```python
from build123d import *

# Parameters (mm, degrees)
SKETCH1_W               = 400
SKETCH1_H               = 200
BOSS_EXTRUDE1_DEPTH     = 52.5
SKETCH2_W               = 400
SKETCH2_H               = 90
CUT_EXTRUDE2_DEPTH      = 40
SKETCH3_W               = 90.375416362
SKETCH3_H               = 10.805756305
CUT_EXTRUDE4_DEPTH      = 30
SKETCH6_W               = 90.866587104
SKETCH6_H               = 12.770439269
CUT_EXTRUDE5_DEPTH      = 30
SKETCH7_W               = 90.866587104
SKETCH7_H               = 151.035002888
CUT_EXTRUDE6_DEPTH      = 416.639567414
SKETCH8_W               = 30
SKETCH8_H               = 90.375416362
CUT_EXTRUDE7_DEPTH      = 256.367226621
SKETCH11_R              = 11.25
CUT_EXTRUDE8_DEPTH      = 248.032386541
FILLET6_R               = 5
CUT_EXTRUDE9_DEPTH      = 248.032386541
CUT_EXTRUDE9_DEPTH_BACK = 248.032386541
SKETCH12_R              = 11.25
FILLET7_R               = 5
SKETCH19_W              = 5.960521718
SKETCH19_H              = 90
CUT_EXTRUDE11_DEPTH     = 262.450282081
SKETCH20_W              = 5
SKETCH20_H              = 90
CUT_EXTRUDE12_DEPTH     = 262.450282081
BOSS_EXTRUDE7_REACH     = 249.032
SKETCH29_W              = 29.604200123
SKETCH29_H              = 5.313574381
SKETCH30_W              = 40.6
SKETCH30_H              = 6.563827177
CUT_EXTRUDE16_DEPTH     = 416.639567414
SKETCH31_R              = 2.65
CUT_EXTRUDE17_DEPTH     = 10
SKETCH32_W              = 53.894825864
SKETCH32_H              = 4.174951299
BOSS_EXTRUDE8_DEPTH     = 5
SKETCH33_W              = 38.657413524
SKETCH33_H              = 4.433580482
BOSS_EXTRUDE9_DEPTH     = 5


with BuildPart() as part:
    # Sketch1 → Boss-Extrude1 (new, symmetric)
    with BuildSketch(Plane.XY):
        Rectangle(SKETCH1_W, SKETCH1_H)
    extrude(amount=BOSS_EXTRUDE1_DEPTH, both=True)

    # Sketch2 → Cut-Extrude2 (cut)
    with BuildSketch(Plane(origin=(0, 100, 0), x_dir=(1, 0, 0), z_dir=(0, 1, 0))):
        Rectangle(SKETCH2_W, SKETCH2_H)
    extrude(amount=-CUT_EXTRUDE2_DEPTH, mode=Mode.SUBTRACT)

    # Sketch3 → Cut-Extrude4 (cut)
    with BuildSketch(Plane(origin=(200, 0, 0), x_dir=(0, 0, -1), z_dir=(1, 0, 0))):
        with Locations((0, 55.256708374)):
            Rectangle(SKETCH3_W, SKETCH3_H)
    extrude(amount=-CUT_EXTRUDE4_DEPTH, mode=Mode.SUBTRACT)

    # Sketch6 → Cut-Extrude5 (cut)
    with BuildSketch(Plane.ZY.offset(200)):
        with Locations((0, 54.274366892)):
            Rectangle(SKETCH6_W, SKETCH6_H)
    extrude(amount=-CUT_EXTRUDE5_DEPTH, mode=Mode.SUBTRACT)

    # Sketch7 → Cut-Extrude6 (cut, through all)
    with BuildSketch(Plane.ZY.offset(200)):
        with Locations((0, -27.628354187)):
            Rectangle(SKETCH7_W, SKETCH7_H)
    extrude(amount=-CUT_EXTRUDE6_DEPTH, mode=Mode.SUBTRACT)

    # Sketch8 → Cut-Extrude7 (cut, through all)
    with BuildSketch(Plane(origin=(0, 49.853830221, 0), x_dir=(1, 0, 0), z_dir=(0, 1, 0))):
        with Locations((185, 0)):
            Rectangle(SKETCH8_W, SKETCH8_H)
    extrude(amount=-CUT_EXTRUDE7_DEPTH, mode=Mode.SUBTRACT)

    # Sketch11 → Cut-Extrude8 (cut, through all)
    with BuildSketch(Plane(origin=(0, 0, -52.5), x_dir=(-1, 0, 0), z_dir=(0, 0, -1))):
        with Locations((-183.256148082, 55.698181941)):
            Circle(SKETCH11_R)
    extrude(amount=-CUT_EXTRUDE8_DEPTH, mode=Mode.SUBTRACT)

    # Fillet6
    fillet6_edges = [part.edges().sort_by_distance(p)[0] for p in [
        (-170, 60, 0),
        (-170, 47.889147257, 0),
    ]]
    fillet(fillet6_edges, radius=FILLET6_R)

    # Sketch12 → Cut-Extrude9 (cut, two sides: drawn at the far end of the back side and taken through both)
    with BuildSketch(Plane.XY.offset(52.5).offset(-CUT_EXTRUDE9_DEPTH_BACK)):
        with Locations((-181.329803839, 56.296045727)):
            Circle(SKETCH12_R)
    extrude(amount=CUT_EXTRUDE9_DEPTH + CUT_EXTRUDE9_DEPTH_BACK, mode=Mode.SUBTRACT)

    # Fillet7
    fillet7_edges = [part.edges().sort_by_distance(p)[0] for p in [
        (170, 47.889147257, 0),
        (170, 60, 0),
    ]]
    fillet(fillet7_edges, radius=FILLET7_R)

    # Sketch19 → Cut-Extrude11 (cut, through all)
    with BuildSketch(Plane(origin=(0, 60, 0), x_dir=(1, 0, 0), z_dir=(0, 1, 0))):
        with Locations((-167.980260859, 0)):
            Rectangle(SKETCH19_W, SKETCH19_H)
    extrude(amount=-CUT_EXTRUDE11_DEPTH, mode=Mode.SUBTRACT)

    # Sketch20 → Cut-Extrude12 (cut, through all)
    with BuildSketch(Plane(origin=(0, 60, 0), x_dir=(1, 0, 0), z_dir=(0, 1, 0))):
        with Locations((167.5, 0)):
            Rectangle(SKETCH20_W, SKETCH20_H)
    extrude(amount=-CUT_EXTRUDE12_DEPTH, mode=Mode.SUBTRACT)

    # Sketch29 → Boss-Extrude7 (add, up to next)
    with BuildSketch(Plane.XY.offset(52.5), mode=Mode.PRIVATE) as boss_extrude7_sk1:
        with Locations((176.486577654, 12.14531287)):
            Rectangle(SKETCH29_W, SKETCH29_H)
    boss_extrude7_tool1 = extrude(boss_extrude7_sk1.sketch, amount=-BOSS_EXTRUDE7_REACH, mode=Mode.PRIVATE) - part.part
    add(boss_extrude7_tool1.solids().sort_by_distance((176.486578, 12.145313, 52.5))[0])

    # Sketch30 → Cut-Extrude16 (cut, through all)
    with BuildSketch(Plane(origin=(200, 0, 0), x_dir=(0, 0, -1), z_dir=(1, 0, 0))):
        with Locations((-1.424009181, 12.770439269)):
            Rectangle(SKETCH30_W, SKETCH30_H)
    extrude(amount=-CUT_EXTRUDE16_DEPTH, mode=Mode.SUBTRACT)

    # Sketch31 → Cut-Extrude17 (cut)
    with BuildSketch(Plane.XY.offset(52.5)):
        with Locations((-94.505715776, 0)):
            Circle(SKETCH31_R)
    extrude(amount=-CUT_EXTRUDE17_DEPTH, mode=Mode.SUBTRACT)

    # Sketch32 → Boss-Extrude8 (add)
    with BuildSketch(Plane.XY.offset(52.5)):
        with Locations((99.43974913, 53.705055351)):
            Rectangle(SKETCH32_W, SKETCH32_H)
    extrude(amount=BOSS_EXTRUDE8_DEPTH)

    # Sketch33 → Boss-Extrude9 (add)
    with BuildSketch(Plane(origin=(0, 0, -52.5), x_dir=(-1, 0, 0), z_dir=(0, 0, -1))):
        with Locations((-111.744568027, 56.347904824)):
            Rectangle(SKETCH33_W, SKETCH33_H)
    extrude(amount=BOSS_EXTRUDE9_DEPTH)


solid = part.part
```
Work out the finished part from the listing and answer in its coordinate system (mm). A direction names the side the tool comes from. Round coordinates to 2 decimals unless told otherwise and drop trailing zeros. Loops run counter-clockwise (first coordinate to the right, second up) from the corner with the lowest first, then second, coordinate; pieces in that order, holes last.
(1) The part is cut by section C-C, the plane x = 18. Give the vertices of the cut face in (y, z), and give its area (3 significant figures).
Computed values:
outline: (-100, -52.5) - (100, -52.5) - (100, -45) - (60, -45) - (60, 45) - (100, 45) - (100, 52.5) - (-100, 52.5) - (-100, 45.43) - (47.89, 45.43) - (47.89, -45.43) - (-100, -45.43) - close
area: 3,960 mm2
(2) Each of these flat-tipped pins is pushed along its axis until it touches: P1, Ø2.5, axis at y = 12, z = 33, coming from the +X side; P2, Ø10, axis at x = -72.5, y = 30, coming from the +Z side; P3, Ø6, axis at x = 57, z = -40.5, coming from the -Y side. Where does it stop, or does it pass through?
Computed values:
P1: stops at x = 191.29
P2: stops at z = 52.5
P3: stops at y = 47.89
(3) The part is cut by section B-B, the plane z = -30.5. Give the vertices of the cut face in (x, y), and give its area (3 significant figures).
Computed values:
outline: (-165, 47.89) - (165, 47.89) - (165, 60) - (-165, 60) - close; (161.68, 9.49) - (191.29, 9.49) - (191.29, 14.8) - (161.68, 14.8) - close
area: 4,150 mm2
(4) The part is cut by section A-A, the plane y = -85.5. Give the vertices of the cut face in (x, z), and give its area (3 significant figures).
Computed values:
outline: (-200, -52.5) - (200, -52.5) - (200, -45.43) - (-200, -45.43) - close; (-200, 45.43) - (200, 45.43) - (200, 52.5) - (-200, 52.5) - close
area: 5,650 mm2
(5) For faces 1 (the flat face through (-200, -1, -49)), 2 (the flat face through (176, 9.489, 34)), 3 (the flat face through (-3, 100, -49)), determine the directions among +Z, -Z, +X, -X, +Y, -Y from which every point of the face is accessible in a straight line to the end or side of a thin tool.
Computed values:
face 1: +Z, -Z, -X, +Y, -Y
face 2: +X, -X, -Y
face 3: +Z, -Z, +X, -X, +Y
(6) Find the intervals of material crossed by L1, parallel to Z at x = -74, y = 35; L2, parallel to Z at x = -11.5, y = 72; L3, parallel to Y at x = 9, z = -44.5, in increasing order.
Computed values:
L1: z = -52.5 to -45.43, 45.43 to 52.5
L2: z = -52.5 to -45, 45 to 52.5
L3: y = 47.89 to 60
(7) The mould has two halves that part along X. Classify faces 4 (the cylindrical face through (-170.6, 59.68, -48.8)), 5 (the flat face through (-2, 60, -1)), 6 (the flat face through (165, 54, 1)): pulls with the +X half, pulls with the -X half, needs draft (parallel to the pull), parting line crosses it, or undercut.
Computed values:
face 4: undercut
face 5: needs draft
face 6: pulls with the +X half
